The listing builds one solid part. Answer for the finished solid, in the listing's coordinates (mm). Face numbers are marked on the shaded views. A direction names the side the tool comes from. Round coordinates to 2 decimals unless told otherwise and drop trailing zeros. Order: outer loops, then holes, each group sorted by start corner. A loop starts at its lowest first (then second) coordinate and runs counter-clockwise, first axis right, second up. Notation, with made-up numbers: M 33.5,23.25 L 64.5,23.25 A20 ccw 64.5,60.25 Z; hole C 31,10 d5. An arc over 180 degrees is marked long. Put each result on its own line as item: value. Start each with the question number.
1. The mould has two halves that part along X. Classify the marked faces 6, 7, 8 and 9: +X half, -X half, draft (parallel to the pull), parting line (faces both ways), or undercut.
2. Each of these flat-tipped pins is pushed along its axis until it touches: pin 1 Ø18 at (x, y) = (-28.5, 45) entering from +Z; pin 2 Ø8 at (x, z) = (-21.5, -31) entering from +Y; pin 3 Ø1 at (x, z) = (13, 55) entering from -Y. Where does it stop, or does it pass through?
3. The part is cut by section A-A (x = 0). Give the vertices of the cut face in (y, z).
4. Which of the six approach directions +Z, -Z, +X, -X, +Y, -Y give full straight-line access (tool end or side, diameter ignored) to the marked faces 1, 2, 3, 4 and 5?
5. The part is cut by section B-B (y = -4). Give the vertices of the cut face in (x, z), then the cut area to 3 significant figures.
6. The part is cut by section C-C (z = -1.5). Give the vertices of the cut face in (x, y).
7. Consider line 1 (X direction, y = 28.5, z = 40.5); line 2 (Z direction, x = 26, y = 26.5); line 3 (X direction, y = 59, z = -23.5). Determine where each line is inside the solid, lowest interval first.
from build123d import *

# Parameters (mm, degrees)
SKETCH2_W           = 200
SKETCH2_H           = 160
BOSS_EXTRUDE1_DEPTH = 10
BOSS_EXTRUDE2_DEPTH = 60
SKETCH8_R           = 12.5
BOSS_EXTRUDE6_DEPTH = 15
FILLET2_R           = 5
CUT_EXTRUDE4_DEPTH  = 15
SKETCH10_R          = 10
CUT_EXTRUDE5_DEPTH  = 10
SKETCH7_R           = 5
CUT_EXTRUDE6_DEPTH  = 10
CUT_EXTRUDE7_DEPTH  = 10
FILLET5_R           = 15


with BuildPart() as part:
    # Sketch2 → Boss-Extrude1 (new body)
    with BuildSketch(Plane(origin=(0, 0, 0), x_dir=(1, 0, 0), z_dir=(0, 1, 0))):
        Rectangle(SKETCH2_W, SKETCH2_H)
    extrude(amount=BOSS_EXTRUDE1_DEPTH)

    # Sketch3 → Boss-Extrude2 (add)
    with BuildSketch(Plane(origin=(0, 10, 0), x_dir=(1, 0, 0), z_dir=(0, 1, 0))):
        Polygon((-100, 80), (100, 80), (100, -80), (60, -80), (60, -20), (-60, -20), (-60, -80), (-100, -80), align=None)
        Polygon((90, 70), (90, -70), (70, -70), (70, -10), (-70, -10), (-70, -70), (-90, -70), (-90, 70), align=None, mode=Mode.SUBTRACT)
    extrude(amount=BOSS_EXTRUDE2_DEPTH)

    # Sketch8 → Boss-Extrude6 (add)
    with BuildSketch(Plane.XZ):
        with Locations(Location((70, 50, 0), (0, 0, 90))):
            Circle(SKETCH8_R)
        with Locations(Location((-70, 50, 0), (0, 0, 90))):
            Circle(SKETCH8_R)
        with Locations(Location((70, -50, 0), (0, 0, 90))):
            Circle(SKETCH8_R)
        with Locations(Location((-70, -50, 0), (0, 0, 90))):
            Circle(SKETCH8_R)
    extrude(amount=BOSS_EXTRUDE6_DEPTH)

    # Fillet2
    fillet2_edges = [part.edges().sort_by_distance(p)[0] for p in [
        (70, -15, 37.5),
        (-70, -15, 37.5),
        (70, -15, -62.5),
        (-70, -15, -62.5),
    ]]
    fillet(fillet2_edges, radius=FILLET2_R)

    # Sketch9 → Cut-Extrude4 (cut)
    with BuildSketch(Plane(origin=(0, 0, -80), x_dir=(-1, 0, 0), z_dir=(0, 0, -1))):
        with BuildLine():
            Line((65, 25), (75, 25))
            ThreePointArc((75, 25), (80, 20), (75, 15))
            Line((75, 15), (65, 15))
            ThreePointArc((65, 15), (60, 20), (65, 25))
        make_face()
    extrude(amount=-CUT_EXTRUDE4_DEPTH, mode=Mode.SUBTRACT)

    # Sketch10 → Cut-Extrude5 (cut)
    with BuildSketch(Plane.XY.offset(80)):
        with Locations((80, 40)):
            Circle(SKETCH10_R)
    extrude(amount=-CUT_EXTRUDE5_DEPTH, mode=Mode.SUBTRACT)

    # Sketch7 → Cut-Extrude6 (cut)
    with BuildSketch(Plane.XY.offset(20)):
        with Locations((0, 25)):
            Circle(SKETCH7_R)
    extrude(amount=-CUT_EXTRUDE6_DEPTH, mode=Mode.SUBTRACT)

    # Sketch11 → Cut-Extrude7 (cut)
    with BuildSketch(Plane.XY.offset(20)):
        with BuildLine():
            Line((47.237449464, 27.403784995), (47.237449464, 17.403784995))
            ThreePointArc((47.237449464, 17.403784995), (44.237449464, 14.403784995), (41.237449464, 17.403784995))
            Line((41.237449464, 17.403784995), (41.237449464, 27.403784995))
            ThreePointArc((41.237449464, 27.403784995), (44.237449464, 30.403784995), (47.237449464, 27.403784995))
        make_face()
    extrude(amount=-CUT_EXTRUDE7_DEPTH, mode=Mode.SUBTRACT)

    # Fillet5
    # the kernel refuses this fillet: 15 mm, written as the material it takes off along each edge
    with BuildSketch(Plane(origin=(-137.5, 0, -80), x_dir=(0, 0, 1), z_dir=(1, 0, 0)), Plane(origin=(137.5, 0, 80), x_dir=(0, 0, -1), z_dir=(-1, 0, 0))) as fillet5_piece_1:
        with BuildLine():
            CenterArc((FILLET5_R, -FILLET5_R), FILLET5_R, 90, 90)
            Line((0, -FILLET5_R), (0, 0))
            Line((0, 0), (FILLET5_R, 0))
        make_face()
    extrude(amount=275, mode=Mode.SUBTRACT)
    with BuildSketch(Plane(origin=(100, 0, -117.5), x_dir=(-1, 0, 0), z_dir=(0, 0, 1)), Plane(origin=(-100, 0, 117.5), x_dir=(1, 0, 0), z_dir=(0, 0, -1))) as fillet5_piece_2:
        with BuildLine():
            CenterArc((FILLET5_R, -FILLET5_R), FILLET5_R, 90, 90)
            Line((0, -FILLET5_R), (0, 0))
            Line((0, 0), (FILLET5_R, 0))
        make_face()
    extrude(amount=235, mode=Mode.SUBTRACT)


solid = part.part
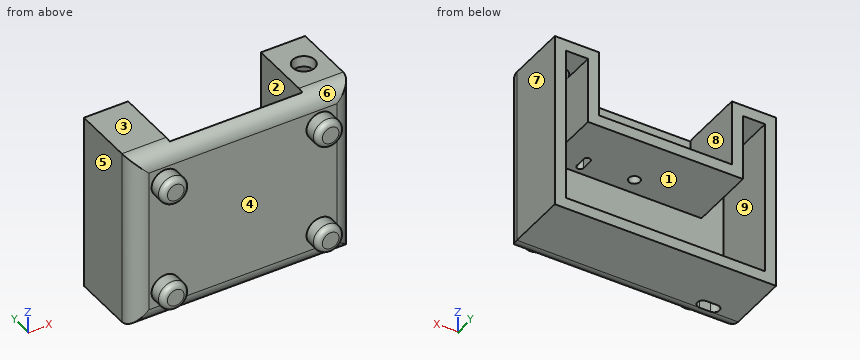
Resolved:
1. face 6: draft
1. face 7: +X half
1. face 8: undercut
1. face 9: undercut
2. pin 1: z = 20
2. pin 2: y = 10
2. pin 3: y = 0
3. outline: M 0,-65 A15 ccw 15,-80 L 70,-80 L 70,-70 L 10,-70 L 10,10 L 20,10 L 20,20 L 10,20 L 10,79.14 A15 ccw 0,65 Z; M 30,10 L 70,10 L 70,20 L 30,20 Z
4. face 1: +Y
4. face 2: +Z, +Y
4. face 3: +Z, +X, -X, +Y, -Y
4. face 4: -Y
4. face 5: +Z, -Z, -X, +Y, -Y
5. outline: C -70,-50 d25; C -70,50 d25; C 70,-50 d25; C 70,50 d25
5. area: 1,960 mm2
6. outline: M -100,15 A15 ccw -85,0 L 85,0 A15 ccw 100,15 L 100,70 L 90,70 L 90,10 L -90,10 L -90,70 L -100,70 Z
7. line 1: -100 to -90, -70 to -60, 60 to 70, 90 to 100
7. line 2: -80 to -70, 10 to 20
7. line 3: -100 to -90, 90 to 100
